Geometry check sheet. Reference: the model listing, model coordinates, mm. Coordinates: 2 decimals unless noted, no trailing zeros. Write each loop counter-clockwise with the first axis right and the second up, starting at its lowest first coordinate (ties: lowest second). Pieces come first, ordered by that corner, then holes. Notation, with made-up numbers: (77.25, 76.5) -> (130.25, 76.5) arc R21 cw to (130.25, 89.5) -> close; hole circle Ø1 at (63, 10.25). An arc over 180 degrees is marked (long way). Use a Markdown table: item, result.
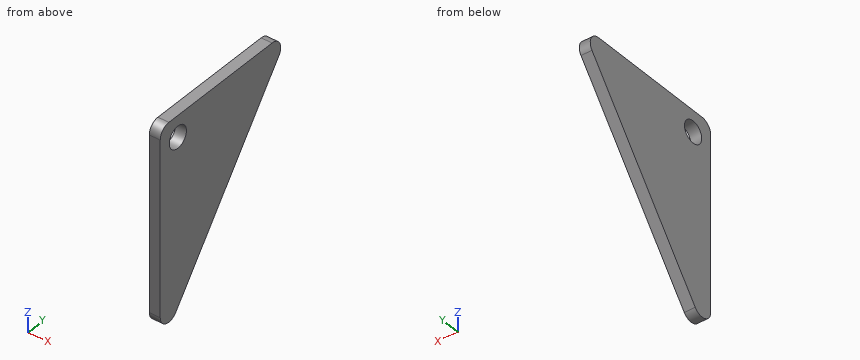
Autodesk Inventor part; units mm, degrees
ref_plane "YZ Plane" through (0, 0, 0) normal (1, 0, 0) x (0, 1, 0)
ref_plane "XZ Plane" through (0, 0, 0) normal (0, 1, 0) x (-1, 0, 0)
ref_plane "XY Plane" through (0, 0, 0) normal (0, 0, 1) x (1, 0, 0)
sketch "Sketch1" plane through (0, 0, 0) normal (1, 0, 0) x (0, 1, 0)
  line L0 (6.712, 10.6489) -> (-8.288, 10.6489)
  line L1 (-8.288, 10.6489) -> (-8.288, -9.3511)
  line L2 (-8.288, -9.3511) -> (6.712, 10.6489)
  point P0 (0, 0)
  dimension "d0" = 20
  dimension "d1" = 15
extrude "Extrusion1" add sketch "Sketch1" along normal blind 1
fillet "Fillet1" radius 1 3 edges at (0.5, 6.712, 10.6489) (0.5, -8.288, 10.6489) (0.5, -8.288, -9.3511)
sketch "Sketch2" plane through (0, 0, 0) normal (-1, 0, 0) x (0, 0, 1)
  point P0 (0, 0)
  point P1 (8.6941, -6.2404)
hole "Hole1" at (0, -6.2404, 8.6941) direction (1, 0, 0) diameter 2 end through all
properties part number "wing_horn"
Item 1: Thickness scan on L1, parallel to Z at x = 0.7, y = 4.5; L2, parallel to Y at x = 0.7, z = 1; L3, parallel to Y at x = 0.75, z = 4.75. Record the ranges inside material, lowest first. Write a range as [from, to].
Answer block:
| item | result |
|---|---|
| L1 | z = [7.7, 10.65] |
| L2 | y = [-8.29, -0.52] |
| L3 | y = [-8.29, 2.29] |
Item 2: Depth check by flat-ended pin: P1, Ø1.5, axis at y = -2, z = -3.5, coming from the +X side (3 decimals); P2, Ø3, axis at y = -6.24, z = 8.69, coming from the -X side. Enter the tip coordinate at first touch or a pass-through.
Answer block:
| item | result |
|---|---|
| P1 | passes through |
| P2 | stops at x = 0 |
Item 3: Section check C-C on x = 0.6. Record the boundary of the cut face in (y, z), then the cut area to 3 significant figures.
Answer block:
| item | result |
|---|---|
| outline | (-8.29, -6.35) arc R1 ccw to (-6.49, -6.95) -> (5.51, 9.05) arc R1 ccw to (4.71, 10.65) -> (-7.29, 10.65) arc R1 ccw to (-8.29, 9.65) -> close; hole circle Ø2 at (-6.24, 8.69) |
| area | 144 mm^2 |
Item 4: Section check A-A on z = 8. Record the boundary of the cut face in (x, y).
Answer block:
| item | result |
|---|---|
| outline | (0, -8.29) -> (1, -8.29) -> (1, -6.96) -> (0, -6.96) -> close; (0, -5.52) -> (1, -5.52) -> (1, 4.73) -> (0, 4.73) -> close |
Item 5: Section check D-D on y = -2.75. Record the boundary of the cut face in (x, z), then the cut area to 3 significant figures.
Answer block:
| item | result |
|---|---|
| outline | (0, -1.97) -> (1, -1.97) -> (1, 10.65) -> (0, 10.65) -> close |
| area | 12.6 mm^2 |
Item 6: Section check B-B on y = -6. Record the boundary of the cut face in (x, z).
Answer block:
| item | result |
|---|---|
| outline | (0, -6.3) -> (1, -6.3) -> (1, 7.72) -> (0, 7.72) -> close; (0, 9.66) -> (1, 9.66) -> (1, 10.65) -> (0, 10.65) -> close |
